Input: part model. Units: mm. Frame: model coordinates. A direction names the side the tool comes from. Round coordinates to 2 decimals unless told otherwise and drop trailing zeros. Order: outer loops, then holes, each group sorted by start corner. A loop starts at its lowest first (then second) coordinate and runs counter-clockwise, first axis right, second up. Notation, with made-up numbers: (75.25, -2) -> (105.25, -2) arc R26 cw to (105.25, 27) -> close; hole circle Ø1 at (83, 48.25). An arc over 180 degrees is marked (long way). Use a Markdown table: item, result.
Autodesk Inventor part; units mm, degrees
ref_plane "YZ Plane" through (0, 0, 0) normal (1, 0, 0) x (0, 1, 0)
ref_plane "XZ Plane" through (0, 0, 0) normal (0, 1, 0) x (-1, 0, 0)
ref_plane "XY Plane" through (0, 0, 0) normal (0, 0, 1) x (1, 0, 0)
sketch "Sketch1" plane through (0, 0, 0) normal (0, 1, 0) x (-1, 0, 0)
  line L0 (0, 0) -> (54.67, 0)
  line L1 (54.67, 0) -> (54.67, -38.1)
  line L2 (54.67, -38.1) -> (0, -38.1)
  line L3 (0, -38.1) -> (0, 0)
  dimension "d0" = 54.67
  dimension "d1" = 38.1
extrude "Extrusion1" add sketch "Sketch1" along normal blind 13.2
sketch "Sketch2" plane through (0, 13.2, 0) normal (0, 1, 0) x (1, 0, 0)
  circle A0 centre (-52.13, 2.54) radius 1.6
  circle A1 centre (-36.25, 2.54) radius 1.6
  circle A2 centre (-4.5, 2.54) radius 1.6
  circle A3 centre (-52.13, 35.56) radius 1.6
  circle A4 centre (-36.25, 35.56) radius 1.6
  circle A5 centre (-4.5, 35.56) radius 1.6
  line L0 (-54.67, 0) -> (0, 0)
  line L1 (0, 38.1) -> (-54.67, 38.1)
  line L2 (-54.67, 38.1) -> (-54.67, 0)
  line L3 (0, 0) -> (0, 38.1)
  dimension "d4" = 3.2
  dimension "d5" = 3.2
  dimension "d6" = 3.2
  dimension "d7" = 3.2
  dimension "d8" = 3.2
  dimension "d9" = 3.2
  dimension "d10" = 2.54
  dimension "d11" = 2.54
  dimension "d12" = 2.54
  dimension "d13" = 2.54
  dimension "d14" = 2.54
  dimension "d15" = 2.54
  dimension "d16" = 2.54
  dimension "d17" = 4.5
  dimension "d18" = 36.25
  dimension "d19" = 4.5
  dimension "d20" = 36.25
  dimension "d21" = 2.54
extrude "Extrusion2" cut sketch "Sketch2" against normal through all contours A0 | A1 | A2 | A3 | A4 | A5
sketch "Sketch3" plane through (0, 13.2, 0) normal (0, 1, 0) x (1, 0, 0)
  arc A0 (-52.13, 31.96) -> (-48.53, 35.56) centre (-52.13, 35.56) ccw
  arc A1 (-39.85, 35.56) -> (-32.65, 35.56) centre (-36.25, 35.56) ccw
  arc A2 (-8.1, 35.56) -> (-2.54, 32.5403) centre (-4.5, 35.56) ccw
  arc A3 (-2.54, 5.5597) -> (-8.1, 2.54) centre (-4.5, 2.54) ccw
  arc A4 (-32.65, 2.54) -> (-39.85, 2.54) centre (-36.25, 2.54) ccw
  arc A5 (-48.53, 2.54) -> (-52.13, 6.14) centre (-52.13, 2.54) ccw
  arc A6 (-52.13, 14.2583) -> (-52.13, 23.8417) centre (-49.43, 19.05) ccw
  line L0 (-48.53, 35.56) -> (-39.85, 35.56)
  line L1 (-32.65, 35.56) -> (-8.1, 35.56)
  line L2 (-2.54, 32.5403) -> (-2.54, 5.5597)
  line L3 (-52.13, 14.2583) -> (-52.13, 6.14)
  line L4 (-48.53, 2.54) -> (-39.85, 2.54)
  line L5 (-32.65, 2.54) -> (-8.1, 2.54)
  line L6 (0, 0) -> (0, 38.1)
  line L7 (0, 38.1) -> (-54.67, 38.1)
  line L8 (-54.67, 0) -> (0, 0)
  line L9 (-54.67, 38.1) -> (-54.67, 0)
  line L10 (-52.13, 31.96) -> (-52.13, 23.8417)
  dimension "d24" = 4.5
  dimension "d25" = 2.54
  dimension "d26" = 2.54
  dimension "d27" = 4.5
  dimension "d28" = 2.54
  dimension "d29" = 36.25
  dimension "d30" = 15.88
  dimension "d31" = 36.25
  dimension "d32" = 15.88
  dimension "d33" = 2.54
  dimension "d34" = 2.54
  dimension "d35" = 2.54
  dimension "d36" = 3.6
  dimension "d37" = 3.6
  dimension "d38" = 3.6
  dimension "d39" = 3.6
  dimension "d40" = 3.6
  dimension "d41" = 3.6
  dimension "d42" = 2.54
  dimension "d43" = 2.54
  dimension "d44" = 2.54
  dimension "d45" = 2.54
  dimension "d46" = 2.54
  dimension "d47" = 2.54
  dimension "d48" = 2.54
  dimension "d49" = 5.24
  dimension "d50" = 19.05
  dimension "d51" = 5.5
extrude "Extrusion3" cut sketch "Sketch3" against normal blind 3 contours A0 L0 A1 L1 A2 L2 A3 L5 A4 L4 A5 L3 A6 L10
sketch "Sketch5" plane through (0, 13.2, 0) normal (0, 1, 0) x (1, 0, 0)
  circle A0 centre (-49.27, 19.05) radius 3.5
  line L0 (-54.67, 38.1) -> (-54.67, 0)
  line L1 (-54.67, 0) -> (0, 0)
  dimension "d61" = 7
  dimension "d62" = 5.4
  dimension "d63" = 19.05
extrude "Extrusion5" cut sketch "Sketch5" against normal blind 0.9
sketch "Sketch15" plane through (-49.27, 12.3, -19.05) normal (0, 1, 0) x (1, 0, 0)
  circle A0 centre (0, 0) radius 2.5
  line L0 (-5.4, 19.05) -> (-5.4, -19.05)
  line L1 (49.27, 19.05) -> (-5.4, 19.05)
  point P0 (49.27, -19.05)
  dimension "d116" = 5
  dimension "d117" = 5.4
  dimension "d118" = 19.05
extrude "Extrusion13" cut sketch "Sketch15" against normal through all
sketch "Sketch18" plane through (0, 0, -38.1) normal (0, 0, -1) x (-1, 0, 0)
  circle A0 centre (49.27, 8.2) radius 1
  line L0 (54.67, 0) -> (54.67, 13.2)
  line L1 (0, 13.2) -> (54.67, 13.2)
  point P0 (0, 0)
  dimension "d124" = 2
  dimension "d125" = 5.4
  dimension "d126" = 5
extrude "Extrusion14" cut sketch "Sketch18" against normal blind 19
sketch "Sketch20" plane through (-54.67, 0, -38.1) normal (-1, 0, 0) x (0, 0, 1)
  line L0 (2, 13.2) -> (0, 13.2)
  line L1 (0, 13.2) -> (0, 12.7)
  line L2 (0, 12.7) -> (2, 12.2)
  line L3 (2, 12.2) -> (2, 13.2)
  point P0 (38.1, 0)
  dimension "d129" = 0.5
  dimension "d130" = 1
  dimension "d131" = 2
extrude "Extrusion15" cut sketch "Sketch20" against normal blind 10.8
sketch "Sketch21" plane through (0, 0, -38.1) normal (0, 0, -1) x (-1, 0, 0)
  circle A0 centre (49.27, 8.2) radius 3.5
  line L0 (54.67, 0) -> (54.67, 12.7)
  line L1 (43.87, 13.2) -> (50.6239, 13.2)
  point P0 (0, 0)
  dimension "d134" = 7
  dimension "d135" = 5.4
  dimension "d136" = 5
extrude "Extrusion16" cut sketch "Sketch21" against normal blind 0.9
properties part number "HousingVX"
1) Cut plane A-A on y = 8.2. Return loops of the section in (x, z), and give its area (3 significant figures).
Results found:
| item | result |
|---|---|
| outline | (-54.67, -38.1) -> (-52.77, -38.1) -> (-52.77, -37.2) -> (-50.27, -37.2) -> (-50.27, -21.34) arc R2.5 cw (long way) to (-48.27, -21.34) -> (-48.27, -37.2) -> (-45.77, -37.2) -> (-45.77, -38.1) -> (0, -38.1) -> (0, 0) -> (-54.67, 0) -> close; hole circle Ø3.2 at (-52.13, -35.56); hole circle Ø3.2 at (-52.13, -2.54); hole circle Ø3.2 at (-36.25, -35.56); hole circle Ø3.2 at (-36.25, -2.54); hole circle Ø3.2 at (-4.5, -35.56); hole circle Ø3.2 at (-4.5, -2.54) |
| area | 1,980 mm² |
2) Pin query (flat end, axial travel): pin 1 Ø3.5 at (x, z) = (-36.25, -2.54) entering from +Y; pin 2 Ø3 at (x, z) = (-4.5, -35.56) entering from +Y; pin 3 Ø2.5 at (x, y) = (-49.27, 8.2) entering from -Z. Return the tip coordinate at first contact, or that it passes through.
Results found:
| item | result |
|---|---|
| pin 1 | stops at y = 13.2 |
| pin 2 | passes through |
| pin 3 | stops at z = -37.2 |
3) Cut plane B-B on x = -4.5. Return loops of the section in (y, z).
Results found:
| item | result |
|---|---|
| outline | (0, -38.1) -> (13.2, -38.1) -> (13.2, -37.16) -> (0, -37.16) -> close; (0, -33.96) -> (13.2, -33.96) -> (13.2, -31.96) -> (10.2, -31.96) -> (10.2, -6.14) -> (13.2, -6.14) -> (13.2, -4.14) -> (0, -4.14) -> close; (0, -0.94) -> (13.2, -0.94) -> (13.2, 0) -> (0, 0) -> close |
4) Cut plane C-C on y = 2.25. Return loops of the section in (x, z).
Results found:
| item | result |
|---|---|
| outline | (-54.67, -38.1) -> (0, -38.1) -> (0, 0) -> (-54.67, 0) -> close; hole circle Ø3.2 at (-52.13, -35.56); hole circle Ø3.2 at (-52.13, -2.54); hole circle Ø5 at (-49.27, -19.05); hole circle Ø3.2 at (-36.25, -35.56); hole circle Ø3.2 at (-36.25, -2.54); hole circle Ø3.2 at (-4.5, -35.56); hole circle Ø3.2 at (-4.5, -2.54) |
5) Pull-direction query (X, two-part tool) for faces 4 (the flat face through (-27, 0, -19)), 5 (the cylindrical face through (-49.6, 11.7, -33)), 6 (the cylindrical face through (-5.77, 6.69, -1.57)), 7 (the flat face through (0, 7, -19)); classes: +X half, -X half, draft (parallel to the pull), parting line (faces both ways), or undercut.
Results found:
| item | result |
|---|---|
| face 4 | draft |
| face 5 | undercut |
| face 6 | undercut |
| face 7 | +X half |
6) Set-up query: faces 1 (the flat face through (-52.13, 12, -28)), 2 (the cylindrical face through (-46.69, 10.565, -37.656)), 3 (the cylindrical face through (-53.4, 6.69, -1.57)). Return all of +Z, -Z, +X, -X, +Y, -Y with unobstructed straight access to the full face (end or side cutting, diameter ignored); none if empty.
Results found:
| item | result |
|---|---|
| face 1 | +Y |
| face 2 | -Z |
| face 3 | +Y, -Y |
7) Cut plane D-D on x = -14. Return loops of the section in (y, z).
Results found:
| item | result |
|---|---|
| outline | (0, -38.1) -> (13.2, -38.1) -> (13.2, -35.56) -> (10.2, -35.56) -> (10.2, -2.54) -> (13.2, -2.54) -> (13.2, 0) -> (0, 0) -> close |
8) Line query: L1, parallel to X at y = 3.5, z = -35.56; L2, parallel to Z at x = -36.25, y = 8.5; L3, parallel to X at y = 12.5, z = -35.5. Output: solid intervals per line, ascending. Write a range as [from, to].
Results found:
| item | result |
|---|---|
| L1 | x = [-54.67, -53.73], [-50.53, -37.85], [-34.65, -6.1], [-2.9, 0] |
| L2 | z = [-38.1, -37.16], [-33.96, -4.14], [-0.94, 0] |
| L3 | x = [-54.67, -53.73], [-50.53, -48.53], [-39.85, -37.85], [-34.65, -32.65], [-8.1, -6.1], [-2.9, 0] |
